Autodesk Inventor part; units mm, degrees
ref_plane "YZ Plane" through (0, 0, 0) normal (1, 0, 0) x (0, 1, 0)
ref_plane "XZ Plane" through (0, 0, 0) normal (0, 1, 0) x (-1, 0, 0)
ref_plane "XY Plane" through (0, 0, 0) normal (0, 0, 1) x (1, 0, 0)
sketch "スケッチ1" plane through (0, 0, 0) normal (0, 0, 1) x (1, 0, 0)
  circle A0 centre (0, 0) radius 2
  circle A1 centre (0, 0) radius 4
  dimension "d0" = 4
  dimension "d1" = 8
extrude "押し出し1" add sketch "スケッチ1" along normal mid plane 185 contours A0 | A1
sketch "スケッチ3" plane through (0, 0, 92.5) normal (0, 0, 1) x (1, 0, 0)
  circle A0 centre (0, 0) radius 2
  dimension "d5" = 4
extrude "押し出し2" cut sketch "スケッチ3" against normal blind 10
sketch "スケッチ4" plane through (0, 0, -92.5) normal (0, 0, -1) x (-1, 0, 0)
  circle A0 centre (0, 0) radius 2
  dimension "d8" = 4
extrude "押し出し3" cut sketch "スケッチ4" against normal blind 10
properties part number "シャフト185mm" material "アルミニウム 7075"
Read the model definition and answer for the solid it produces. Units are mm, in the model's axes. A direction names the side the tool comes from. Round coordinates to 2 decimals unless told otherwise and drop trailing zeros. Write each loop counter-clockwise with the first axis right and the second up, starting at its lowest first coordinate (ties: lowest second). Pieces come first, ordered by that corner, then holes. Notation, with made-up numbers: (23.25, 17) -> (38.25, 17) arc R23 cw to (38.25, 28) -> close; hole circle Ø4 at (5.25, 13). An arc over 180 degrees is marked (long way). Answer in a Markdown table with one row per item. Add a question column.
1) Which of the six approach directions +Z, -Z, +X, -X, +Y, -Y give full straight-line access (tool end or side, diameter ignored) to faces 5 (the face through (0, 0, -82.5)), 6 (the face through (0, 0, 82.5)), 7 (the face through (-2, -1, 92.5))?
2) Find section C-C, the plane z = 40. Determine the outline of the cut face in (x, y).
3) Find section A-A, the plane x = 0. Determine the outline of the cut face in (y, z), and give its area (3 significant figures).
4) Given P1, Ø2.5, axis at x = 0, y = 0, coming from the +Z side; P2, Ø2, axis at y = 3, z = -41.5, coming from the -X side; P3, Ø2, axis at x = 3, z = -41.5, coming from the +Y side, each flat-ended and moving along its own axis, determine where each tip first touches the part or whether it passes through.
5) Determine the mould class of faces 1 (the face through (-2, -1, -92.5)), 2 (the face through (0, -2, 88)), 3 (the face through (-0.867, -3.905, 1.295)), 4 (the face through (0, -2, -88)) for opening direction Y: pulls with the +Y half, pulls with the -Y half, needs draft (parallel to the pull), parting line crosses it, or undercut.
6) Consider line 1 (Y direction, x = 0, z = -86.75); line 2 (X direction, y = -0.25, z = -83); line 3 (Z direction, x = 0, y = -0.5). Determine where each line is inside the solid, lowest interval first.
Findings below:
| question | item | result |
|---|---|---|
| 1 | face 5 | -Z |
| 1 | face 6 | +Z |
| 1 | face 7 | +Z, +X, -X, +Y, -Y |
| 2 | outline | circle Ø8 at (0, 0) |
| 3 | outline | (-4, -92.5) -> (-2, -92.5) -> (-2, -82.5) -> (2, -82.5) -> (2, -92.5) -> (4, -92.5) -> (4, 92.5) -> (2, 92.5) -> (2, 82.5) -> (-2, 82.5) -> (-2, 92.5) -> (-4, 92.5) -> close |
| 3 | area | 1,400 mm² |
| 4 | P1 | z = 82.5 |
| 4 | P2 | x = -3.46 |
| 4 | P3 | y = 3.46 |
| 5 | face 1 | needs draft |
| 5 | face 2 | undercut |
| 5 | face 3 | parting line crosses it |
| 5 | face 4 | undercut |
| 6 | line 1 | -4 to -2, 2 to 4 |
| 6 | line 2 | -3.99 to -1.98, 1.98 to 3.99 |
| 6 | line 3 | -82.5 to 82.5 |
